Could you check a few things on this model? Use its own coordinates, in mm. Give positions to 0.01 mm unless a question says otherwise; leave off trailing zeros. Write each loop counter-clockwise with the first axis right and the second up, starting at its lowest first coordinate (ties: lowest second). Pieces come first, ordered by that corner, then holes. Notation, with made-up numbers: (1, 82) -> (27, 82) arc R22 cw to (27, 99) -> close; hole circle Ø1 at (-8.5, -25). An arc over 180 degrees is marked (long way). One line per question, with ' | ' between items.
from build123d import *

# Parameters (mm, degrees)
F1_DEPTH = 12.7
F2_R     = 5.08
F3_R     = 1


with BuildPart() as f1:
    # F0 (on Front) → F1 (new body)
    with BuildSketch(Plane.XZ):
        Polygon((-11.409408, 1.629178), (-11.409408, -49.170822), (3.830592, -49.170822), (3.830592, 1.629178), (1.432159, 5.782014), (0, 5.782014), (-8.4836, 5.782014), align=None)
    extrude(amount=F1_DEPTH)

    # F2
    f2_edges = [f1.edges().sort_by_distance(p)[0] for p in [
        (-11.409408, 0, -23.770822),
        (-11.409408, -12.7, -23.770822),
        (3.830592, -12.7, -23.770822),
        (3.830592, 0, -23.770822),
    ]]
    fillet(f2_edges, radius=F2_R)

    # F3
    f3_edges = [f1.edges().sort_by_distance(p)[0] for p in [
        (1.432159, -6.35, 5.782014),
        (-8.4836, -6.35, 5.782014),
    ]]
    fillet(f3_edges, radius=F3_R)


solid = f1.part
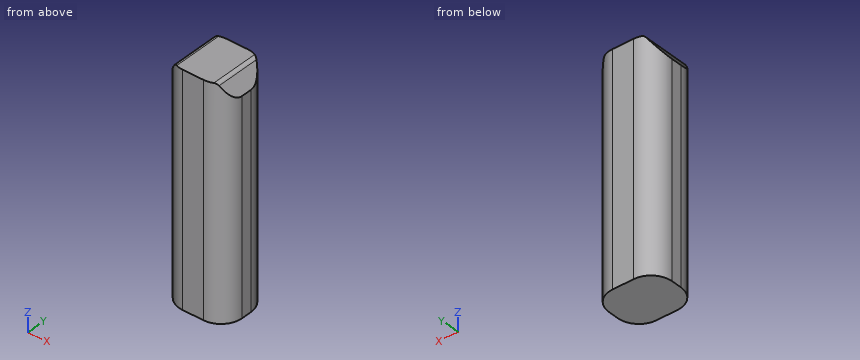
Q1. Imagine slicing it at B-B on z = -4.5. Please give me the cut outline in (x, y).
Answer below:
outline: (-11.41, -7.62) arc R5.08 ccw to (-6.33, -12.7) -> (-1.25, -12.7) arc R5.08 ccw to (3.83, -7.62) -> (3.83, -5.08) arc R5.08 ccw to (-1.25, 0) -> (-6.33, 0) arc R5.08 ccw to (-11.41, -5.08) -> close
Q2. Imagine slicing it at C-C on x = -10. Please give me the cut outline in (y, z), and give its area (3 significant figures).
Answer below:
outline: (-11.13, -49.17) -> (-1.57, -49.17) -> (-1.57, 3.63) -> (-11.13, 3.63) -> close | area: 505 mm^2
Q3. Imagine slicing it at A-A on y = -1.75. Please give me the cut outline in (x, z), and give its area (3 significant figures).
Answer below:
outline: (-10.17, -49.17) -> (2.59, -49.17) -> (2.59, 3.78) -> (1.72, 5.28) arc R1 ccw to (0.85, 5.78) -> (-7.96, 5.78) arc R1 ccw to (-8.78, 5.36) -> (-10.17, 3.39) -> close | area: 698 mm^2
Q4. If I drill on line 1 along X through (y, z) = (-5, -47); line 2 along Y through (x, z) = (-7.25, -3.5); line 3 along X through (y, z) = (-1.75, 3), over which ranges is the centre line in solid material (lowest first)?
Answer below:
line 1: x = -11.41 to 3.83 | line 2: y = -12.62 to -0.08 | line 3: x = -10.17 to 2.59
